Could you check a few things on this model? Use its own coordinates, in mm. Face numbers are marked on the shaded views. A direction names the side the tool comes from. Coordinates: 2 decimals unless noted, no trailing zeros. Order: outer loops, then holes, each group sorted by start corner. A loop starts at its lowest first (then second) coordinate and runs counter-clockwise, first axis right, second up. Notation, with made-up numbers: (65.5, -36) - (94.5, -36) arc R33 ccw to (94.5, -1) - close; hole circle Ø8 at (59.25, -7.5). An arc over 180 degrees is marked (long way). One line per item, written item: value.
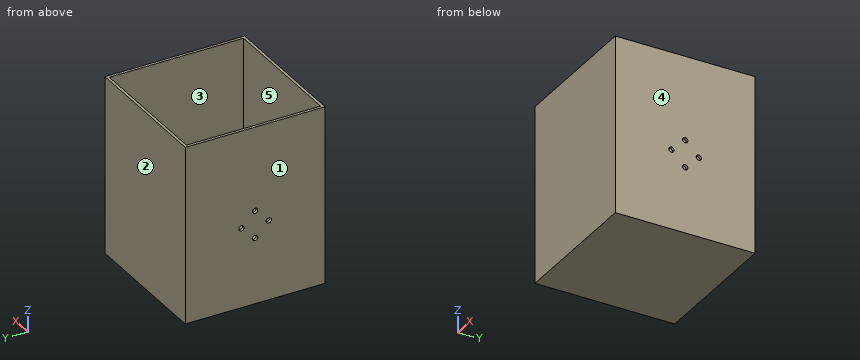
from build123d import *

# Parameters (mm, degrees)
SKETCH1_W               = 100
SKETCH1_H               = 100
BOSS_EXTRUDE2_DEPTH     = 2
SKETCH2_W               = 100
SKETCH2_H               = 100
SKETCH2_W_2             = 96
SKETCH2_H_2             = 96
BOSS_EXTRUDE4_DEPTH     = 125
CUT_EXTRUDE1_DEPTH      = 196.282511518
CUT_EXTRUDE1_DEPTH_BACK = 196.282511518
SKETCH3_R               = 1.9


with BuildPart() as part:
    # Sketch1 → Boss-Extrude2 (new body)
    with BuildSketch(Plane.XY):
        with Locations((119.248829914, 59.573077464)):
            Rectangle(SKETCH1_W, SKETCH1_H)
    extrude(amount=BOSS_EXTRUDE2_DEPTH)

    # Sketch2 → Boss-Extrude4 (add)
    with BuildSketch(Plane.XY.offset(2)):
        with Locations((119.248829914, 59.573077464)):
            Rectangle(SKETCH2_W, SKETCH2_H)
        with Locations((119.248829914, 59.573077464)):
            Rectangle(SKETCH2_W_2, SKETCH2_H_2, mode=Mode.SUBTRACT)
    extrude(amount=BOSS_EXTRUDE4_DEPTH)

    # Sketch3 → Cut-Extrude1 (cut, two sides: drawn at the far end of the back side and taken through both)
    with BuildSketch(Plane(origin=(169.248829914, 0, 0), x_dir=(0, 0, -1), z_dir=(1, 0, 0)).offset(-CUT_EXTRUDE1_DEPTH_BACK)):
        with Locations(Location((-57, 69.352077464, 0), (0, 0, 270))):
            Circle(SKETCH3_R)
        with Locations(Location((-47.221, 59.573077464, 0), (0, 0, 270))):
            Circle(SKETCH3_R)
        with Locations(Location((-57, 49.794077464, 0), (0, 0, 270))):
            Circle(SKETCH3_R)
        with Locations(Location((-66.779, 59.573077464, 0), (0, 0, 270))):
            Circle(SKETCH3_R)
    extrude(amount=CUT_EXTRUDE1_DEPTH + CUT_EXTRUDE1_DEPTH_BACK, mode=Mode.SUBTRACT)


solid = part.part
Item 1: I want a section at B-B on z = 97.5. Please give me the cut outline in (x, y), then the cut area to 3 significant figures.
Conclusion:
outline: (69.25, 9.57) - (169.25, 9.57) - (169.25, 109.57) - (69.25, 109.57) - close; hole (71.25, 11.57) - (167.25, 11.57) - (167.25, 107.57) - (71.25, 107.57) - close
area: 784 mm²
Item 2: I want a section at C-C on y = 84. Please give me the cut outline in (x, z).
Conclusion:
outline: (69.25, 0) - (169.25, 0) - (169.25, 127) - (167.25, 127) - (167.25, 2) - (71.25, 2) - (71.25, 127) - (69.25, 127) - close
Item 3: I want a section at A-A on z = 57. Please give me the cut outline in (x, y).
Conclusion:
outline: (69.25, 9.57) - (169.25, 9.57) - (169.25, 47.89) - (167.25, 47.89) - (167.25, 11.57) - (71.25, 11.57) - (71.25, 47.89) - (69.25, 47.89) - close; (69.25, 51.69) - (71.25, 51.69) - (71.25, 67.45) - (69.25, 67.45) - close; (69.25, 71.25) - (71.25, 71.25) - (71.25, 107.57) - (167.25, 107.57) - (167.25, 71.25) - (169.25, 71.25) - (169.25, 109.57) - (69.25, 109.57) - close; (167.25, 51.69) - (169.25, 51.69) - (169.25, 67.45) - (167.25, 67.45) - close
Item 4: If I drill on probe 1 along X at (y, z) = (76.5, 81); probe 2 along Y at (x, z) = (154.5, 83.5); probe 3 along Z at (x, y) = (123, 80), over which ranges is the centre line in solid material (lowest first)?
Conclusion:
probe 1: 69.25 to 71.25, 167.25 to 169.25
probe 2: 9.57 to 11.57, 107.57 to 109.57
probe 3: 0 to 2
Item 5: For the marked faces 4 and 5, which set-ups out of +Z, -Z, +X, -X, +Y, -Y let a thin tool reach every point of the face, with its end or its side?
Conclusion:
face 4: +Z, -Z, +X, +Y, -Y
face 5: +Z
Item 6: Thinking about a two-plate mould opening in X: for the marked faces 1, 2 and 3, which applies, pulls with the +X half, pulls with the -X half, needs draft (parallel to the pull), parting line crosses it, or undercut?
Conclusion:
face 1: pulls with the -X half
face 2: needs draft
face 3: undercut
Item 7: I'm going to push flat-ended pins straight in: pin 1 Ø5 at (y, z) = (49.79, 57) entering from -X; pin 2 Ø1.5 at (x, y) = (132, 59.5) entering from +Z. Where does each tip first touch, or does it pass through?
Conclusion:
pin 1: x = 69.25
pin 2: z = 2
